The model under review builds one solid part; all positions refer to its coordinate system, in mm. A direction names the side the tool comes from. Round coordinates to 2 decimals unless told otherwise and drop trailing zeros. Write each loop counter-clockwise with the first axis right and the second up, starting at its lowest first coordinate (ties: lowest second). Pieces come first, ordered by that corner, then holes. Notation, with made-up numbers: M 3,27.25 L 30,27.25 A13 ccw 30,46.25 Z; hole C 52.5,72.5 d6. An arc over 180 degrees is marked long. Write item = value, one per line. Start each with the question number.
Item 1: Take a section at B-B, the plane z = 0. Give the boundary of the cut face in (x, y) (3 decimals).
Item 2: Take a section at C-C, the plane y = 34. Give the boundary of the cut face in (x, z), plus the area to 3 significant figures.
Item 3: To check wall thickness, follow line 1 along X through (y, z) = (12.5, -0.5); line 2 along Z through (x, y) = (10, 17); line 3 along X through (y, z) = (10, 5). State the ranges of each line that lie inside material, in increasing order.
Item 4: Take a section at A-A, the plane x = 0. Give the boundary of the cut face in (y, z) (3 decimals).
Item 5: The part is to be moulded in two halves that separate along Z. For faces 1 (the flat face through (6, 0, 5)), 2 (the cylindrical face through (-15.456, 25.055, -20.157)), 3 (the cylindrical face through (-2.75, 28.85, -12.4)), 4 (the cylindrical face through (-0.83, 4.27, 6.31)), say which applies: +Z half, -Z half, draft (parallel to the pull), parting line (faces both ways), or undercut.
Item 6: For pin 1 Ø4 at (x, y) = (14, 18.5) entering from -Z; pin 2 Ø23 at (x, z) = (0, 0) entering from +Y; pin 3 Ø2 at (y, z) = (18.5, -1) entering from +X; pin 4 Ø7.5 at (x, z) = (0, 0) entering from +Y, all flat-tipped, find the tip position at first contact; note any pin that passes through.
Item 7: Tool access review of faces 5 (the flat face through (-11, 50.8, 11)), 6 (the flat face through (-6, 7.874, 3)): name each direction out of +Z, -Z, +X, -X, +Y, -Y from which nothing blocks a thin tool from reaching the whole face with its end or side.
from build123d import *

# Parameters (mm, degrees)
SKETCH1_R                  = 25.4
EXTRUDE1_DEPTH             = 50.8
F_1_2_0_5_DIAMETER_HOLE1_D = 12.7254
CHAMFER1_SIZE              = 0.762
F_1_1_DIAMETER_HOLE1_D     = 25.4
F_1_1_DIAMETER_HOLE1_DEPTH = 42.926
CHAMFER2_SIZE              = 0.254
CHAMFER3_SIZE              = 0.635


with BuildPart() as part:
    # Sketch1 → Extrude1 (new body)
    with BuildSketch(Plane(origin=(0, 0, 0), x_dir=(1, 0, 0), z_dir=(0, 1, 0))):
        with Locations(Location((0, 0, 0), (0, 0, 270))):  # turned: the seam where the file's is
            Circle(SKETCH1_R)
    extrude(amount=EXTRUDE1_DEPTH)

    # 1/2 (0.5) Diameter Hole1 (through all)
    with Locations(Plane(origin=(0, 50.8, 0), x_dir=(-1, 0, 0), z_dir=(0, 1, 0))):
        with Locations((0, 0)):
            Hole(F_1_2_0_5_DIAMETER_HOLE1_D / 2)

    # Chamfer1
    chamfer1_edges = [part.edges().sort_by_distance(p)[0] for p in [
        (0, 0, -25.4),
        (0, 50.8, -25.4),
        (-6.3627, 0, 0),
    ]]
    chamfer(chamfer1_edges, length=CHAMFER1_SIZE)

    # 1 (1) Diameter Hole1
    with Locations(Plane(origin=(0, 50.8, 0), x_dir=(-1, 0, 0), z_dir=(0, 1, 0))):
        with Locations((0, 0)):
            Hole(F_1_1_DIAMETER_HOLE1_D / 2, depth=F_1_1_DIAMETER_HOLE1_DEPTH)

    # Chamfer2
    chamfer2_edges = [part.edges().sort_by_distance(p)[0] for p in [
        (-12.7, 7.874, 0),
    ]]
    chamfer(chamfer2_edges, length=CHAMFER2_SIZE)

    # Chamfer3
    chamfer3_edges = [part.edges().sort_by_distance(p)[0] for p in [
        (-12.7, 50.8, 0),
    ]]
    chamfer(chamfer3_edges, length=CHAMFER3_SIZE)


solid = part.part
Response values:
q1.outline = M -25.4,0.762 L -24.638,0 L -7.125,0 L -6.363,0.762 L -6.363,7.874 L -12.446,7.874 L -12.7,8.128 L -12.7,50.165 L -13.335,50.8 L -24.638,50.8 L -25.4,50.038 Z; M 6.363,0.762 L 7.125,0 L 24.638,0 L 25.4,0.762 L 25.4,50.038 L 24.638,50.8 L 13.335,50.8 L 12.7,50.165 L 12.7,8.128 L 12.446,7.874 L 6.363,7.874 Z
q2.outline = C 0,0 d50.8; hole C 0,0 d25.4
q2.area = 1,520 mm2
q3.line_1 = -25.4 to -12.69, 12.69 to 25.4
q3.line_2 = -23.35 to -7.83, 7.83 to 23.35
q3.line_3 = -24.9 to -11.67, 11.67 to 24.9
q4.outline = M 0,-24.638 L 0.762,-25.4 L 50.038,-25.4 L 50.8,-24.638 L 50.8,-13.335 L 50.165,-12.7 L 8.128,-12.7 L 7.874,-12.446 L 7.874,-6.363 L 0.762,-6.363 L 0,-7.125 Z; M 0,7.125 L 0.762,6.363 L 7.874,6.363 L 7.874,12.446 L 8.128,12.7 L 50.165,12.7 L 50.8,13.335 L 50.8,24.638 L 50.038,25.4 L 0.762,25.4 L 0,24.638 Z
q5.face_1 = draft
q5.face_2 = parting line
q5.face_3 = undercut
q5.face_4 = undercut
q6.pin_1 = -22.39
q6.pin_2 = 7.87
q6.pin_3 = 25.4
q6.pin_4 = through
q7.face_5 = +Z, -Z, +X, -X, +Y
q7.face_6 = +Y
